from build123d import *

# Parameters (mm, degrees)
F0_W      = 44
F0_H      = 45
F1_DEPTH  = 10
F2_R      = 1.25
F3_DEPTH  = 88.001
F4_SIZE   = 0.5
F5_W      = 3
F5_H      = 20
F6_DEPTH  = 10
F7_R      = 1.65
F8_DEPTH  = 10.001
F9_SIZE   = 0.75
F10_R     = 1.25
F11_DEPTH = 15
F12_SIZE  = 0.5


with BuildPart() as f1:
    # F0 (on Top) → F1 (new body)
    with BuildSketch(Plane.XY):
        with Locations((-22, 22.5)):
            Rectangle(F0_W, F0_H)
        with Locations((22, 22.5)):
            Rectangle(F0_W, F0_H)
    extrude(amount=F1_DEPTH)

    # F2 (on face) → F3 (cut, through all)
    with BuildSketch(Plane(origin=(-44, 0, 0), x_dir=(0, -1, 0), z_dir=(-1, 0, 0))):
        with Locations((-21, 7)):
            Circle(F2_R)
        with Locations((-11, 7)):
            Circle(F2_R)
    extrude(amount=-F3_DEPTH, mode=Mode.SUBTRACT)

    # F4
    f4_edges = [f1.edges().sort_by_distance(p)[0] for p in [
        (-44, 22.25, 7),
        (-44, 12.25, 7),
        (44, 12.25, 7),
        (44, 22.25, 7),
    ]]
    chamfer(f4_edges, length=F4_SIZE)

    # F5 (on face) → F6 (join, through all)
    with BuildSketch(Plane.XY.offset(10)):
        with Locations((-45.5, 35)):
            Rectangle(F5_W, F5_H)
        with Locations((45.5, 35)):
            Rectangle(F5_W, F5_H)
    extrude(amount=-F6_DEPTH)

    # F7 (on face) → F8 (cut, through all)
    with BuildSketch(Plane.XY.offset(10)):
        with BuildLine():
            Line((0, 31.125), (0, 37.875))
            ThreePointArc((0, 37.875), (-3.375, 34.5), (0, 31.125))
        make_face()
        with BuildLine():
            ThreePointArc((0, 31.125), (2.3864853865, 32.1135146135), (3.375, 34.5))
            ThreePointArc((3.375, 34.5), (2.3864853865, 36.8864853865), (0, 37.875))
            Line((0, 37.875), (0, 31.125))
        make_face()
        with Locations((-34.5, 38.35)):
            Circle(F7_R)
        with BuildLine():
            ThreePointArc((-17.85, 38.35), (-19.5, 40), (-21.15, 38.35))
            ThreePointArc((-21.15, 38.35), (-19.5, 36.7), (-17.85, 38.35))
        make_face()
        with Locations((19.5, 38.35)):
            Circle(F7_R)
        with BuildLine():
            ThreePointArc((36.15, 38.35), (34.5, 40), (32.85, 38.35))
            ThreePointArc((32.85, 38.35), (34.5, 36.7), (36.15, 38.35))
        make_face()
    extrude(amount=-F8_DEPTH, mode=Mode.SUBTRACT)

    # F9
    f9_edges = [f1.edges().sort_by_distance(p)[0] for p in [
        (0, 37.875, 10),
        (0, 37.875, 0),
        (-36.15, 38.35, 10),
        (-17.85, 38.35, 10),
        (17.85, 38.35, 10),
        (36.15, 38.35, 10),
        (36.15, 38.35, 0),
        (17.85, 38.35, 0),
        (-17.85, 38.35, 0),
        (-36.15, 38.35, 0),
    ]]
    chamfer(f9_edges, length=F9_SIZE)

    # F10 (on face) → F11 (cut)
    with BuildSketch(Plane(origin=(0, 45, 0), x_dir=(-1, 0, 0), z_dir=(0, 1, 0))):
        with Locations((-42, 4.9999999996)):
            Circle(F10_R)
        with Locations((42, 4.9999999996)):
            Circle(F10_R)
        with Locations((-27, 4.9999999996)):
            Circle(F10_R)
        with Locations((-12, 4.9999999996)):
            Circle(F10_R)
        with Locations((12, 4.9999999996)):
            Circle(F10_R)
        with Locations((27, 4.9999999996)):
            Circle(F10_R)
    extrude(amount=-F11_DEPTH, mode=Mode.SUBTRACT)

    # F12
    f12_edges = [f1.edges().sort_by_distance(p)[0] for p in [
        (43.25, 45, 5),
        (-40.75, 45, 5),
        (28.25, 45, 5),
        (13.25, 45, 5),
        (-10.75, 45, 5),
        (-25.75, 45, 5),
    ]]
    chamfer(f12_edges, length=F12_SIZE)


solid = f1.part
For this review, take the finished solid that the model builds, in its own axes (mm). A direction names the side the tool comes from. Round coordinates to 2 decimals unless told otherwise and drop trailing zeros. Write each loop counter-clockwise with the first axis right and the second up, starting at its lowest first coordinate (ties: lowest second). Pieces come first, ordered by that corner, then holes. Notation, with made-up numbers: (65.25, 38.25) -> (89.25, 38.25) arc R22 ccw to (89.25, 49.25) -> close; hole circle Ø7 at (49.5, -3.5). An arc over 180 degrees is marked (long way). Put each result on its own line as item: value.
Q1. Clearance check with flat-ended pins moving along their axes: pin 1 Ø2.5 at (x, y) = (19.5, 38.35) entering from +Z; pin 2 Ø0.8 at (x, z) = (26.5, 5) entering from +Y; pin 3 Ø1.5 at (x, z) = (45.5, 7.5) entering from -Y; pin 4 Ø3 at (y, z) = (11, 7) entering from +X. State where each tip first meets the part, or that it passes through.
Determined:
pin 1: passes through
pin 2: stops at y = 30
pin 3: stops at y = 25
pin 4: stops at x = 43.75
Q2. To check wall thickness, follow L1, parallel to Y at x = 13, z = 7.75; L2, parallel to Z at x = -15.5, y = 11; L3, parallel to Y at x = -34.5, z = 3. State the ranges of each line that lie inside material, in increasing order. Write a range as [from, to].
Determined:
L1: y = [0, 10], [12, 20], [22, 45]
L2: z = [0, 5.75], [8.25, 10]
L3: y = [0, 36.7], [40, 45]
Q3. The part is to be moulded in two halves that separate along Z. For faces 4 (the flat face through (12, 30, 5)), 5 (the flat face through (-42, 30, 5)), 6 (the flat face through (-1, 23, 10)), 7 (the flat face through (-1, 0, 5)), say which applies: released by +Z, released by -Z, zero draft, split by the parting line, or undercut.
Determined:
face 4: undercut
face 5: undercut
face 6: released by +Z
face 7: zero draft
Q4. Consider section B-B on x = 24. State the section outline as (y, z) points, and give its area (3 significant figures).
Determined:
outline: (0, 0) -> (45, 0) -> (45, 10) -> (0, 10) -> close; hole circle Ø2.5 at (11, 7); hole circle Ø2.5 at (21, 7)
area: 440 mm^2
Q5. Consider section C-C on x = 1. Give the number of separate pieces and of enclosed holes in the cut face, and give its area (3 significant figures).
Determined:
separate pieces: 2
enclosed holes: 2
area: 375 mm^2
Q6. Consider section A-A on x = -34.5. State the section outline as (y, z) points.
Determined:
outline: (0, 0) -> (35.95, 0) -> (36.7, 0.75) -> (36.7, 9.25) -> (35.95, 10) -> (0, 10) -> close; (40, 0.75) -> (40.75, 0) -> (45, 0) -> (45, 10) -> (40.75, 10) -> (40, 9.25) -> close; hole circle Ø2.5 at (11, 7); hole circle Ø2.5 at (21, 7)
Q7. Machinability: for faces 1 (the cylindrical face through (-28.155, 37.352, 4.521)), 2 (the flat face through (-44, 12, 5)), 3 (the flat face through (47, 35, 5)), which of the approach directions +Z, -Z, +X, -X, +Y, -Y give a long, thin tool a straight path to every point of the face, cutting with its end or side? Answer none if there is none.
Determined:
face 1: +Y
face 2: +Z, -Z, -X, -Y
face 3: +Z, -Z, +X, +Y, -Y
